```python
from build123d import *

# Parameters (mm, degrees)
SKETCH2_R           = 30
BOSS_EXTRUDE1_DEPTH = 8


with BuildPart() as part:
    # Sketch1 → Revolve1 (revolve)
    with BuildSketch(Plane.XY):
        with BuildLine():
            Line((0, 0), (25, 0))
            Line((25, 0), (25, 11.42377433))
            ThreePointArc((25, 11.42377433), (23.792992012, 18.861807529), (24.672326333, 26.345655289))
            ThreePointArc((24.672326333, 26.345655289), (25.273083835, 32.826746989), (23.760908087, 39.157527645))
            Line((23.760908087, 39.157527645), (15.581247413, 58.617194357))
            Line((15.581247413, 58.617194357), (13.5, 60))
            Line((13.5, 60), (0, 60))
            Line((0, 60), (0, 0))
        make_face()
    revolve(axis=Axis((0, 0, 0), (0, -1, 0)))

    # Sketch2 → Boss-Extrude1 (add)
    with BuildSketch(Plane.XZ):
        Circle(SKETCH2_R)
    extrude(amount=BOSS_EXTRUDE1_DEPTH)


solid = part.part
```
Part model, mm, in its own coordinate system. A direction names the side the tool comes from. Round coordinates to 2 decimals unless told otherwise and drop trailing zeros. Write each loop counter-clockwise with the first axis right and the second up, starting at its lowest first coordinate (ties: lowest second). Pieces come first, ordered by that corner, then holes.
Item 1: Drop flat-ended pins along their axis: pin 1 Ø5 at (x, z) = (-19.5, -23) entering from +Y; pin 2 Ø5 at (x, y) = (-14, 39.5) entering from -Z; pin 3 Ø10 at (x, y) = (-14, 1.5) entering from +Z. Give the stop position or say it passes through.
Results:
pin 1: stops at y = 0
pin 2: stops at z = -21.02
pin 3: stops at z = 28.54
Item 2: Cut at B-B, the plane y = 49.5. Give the cut face in (x, z), plus the area to 3 significant figures.
Results:
outline: circle Ø38.83 at (0, 0)
area: 1,180 mm2
Item 3: Cut at A-A, the plane y = 18.5. Give the cut face in (x, z), plus the area to 3 significant figures.
Results:
outline: circle Ø47.61 at (0, 0)
area: 1,780 mm2
Item 4: Probe L1, parallel to X at y = 17.5, z = 2; L2, parallel to Y at x = 2, z = -25.5; L3, parallel to X at y = 31, z = -5. List the from-to ranges inside material, lowest first.
Results:
L1: x = -23.77 to 23.77
L2: y = -8 to 0
L3: x = -24.82 to 24.82
Item 5: Which spindle directions (+Z, -Z, +X, -X, +Y, -Y) get a long thin tool onto all of the face, cutting with end or side? Do faces 1 (the cylindrical face through (-29.97, -3.94, 1.32)), 2 (the cylindrical face through (23.846, 5.792, 7.509)). Say none if no direction does.
Results:
face 1: +Y, -Y
face 2: none
